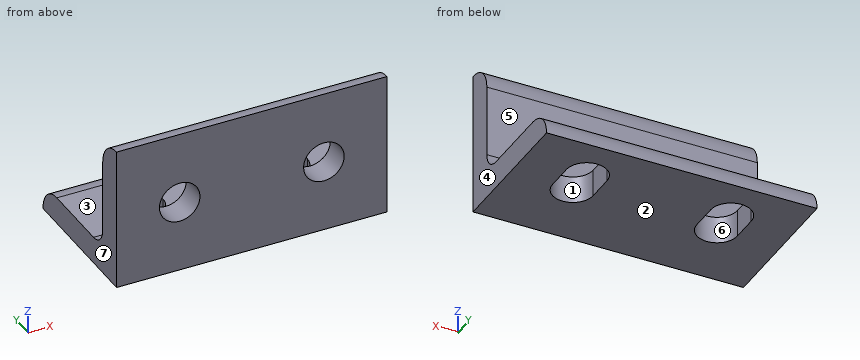
Autodesk Inventor part; units mm, degrees
ref_plane "YZ Plane" through (0, 0, 0) normal (1, 0, 0) x (0, 1, 0)
ref_plane "XZ Plane" through (0, 0, 0) normal (0, 1, 0) x (-1, 0, 0)
ref_plane "XY Plane" through (0, 0, 0) normal (0, 0, 1) x (1, 0, 0)
sketch "Sketch_1" plane through (0, 0, 0) normal (1, 0, 0) x (0, 1, 0)
  line L0 (0, 25.4) -> (0, 0)
  line L1 (0, 0) -> (25.4, 0)
  arc A0 (25.4, 0) -> (20.6248, 4.7752) centre (20.6248, 0) ccw
  line L2 (20.6248, 4.7752) -> (7.9502, 4.7752)
  arc A1 (4.7752, 7.9502) -> (7.9502, 4.7752) centre (7.9502, 7.9502) ccw
  line L3 (4.7752, 7.9502) -> (4.7752, 20.6248)
  arc A2 (4.7752, 20.6248) -> (0, 25.4) centre (0, 20.6248) ccw
extrude "Extrusion1" add sketch "Sketch_1" along normal mid plane 47.625
sketch "Sketch2" plane through (-23.8125, 0, 0) normal (0, -1, 0) x (1, 0, 0)
  point P0 (36.5125, 12.7)
hole "Hole1" at (12.7, 0, 12.7) direction (0, 1, 0) diameter 7.1374 depth 10.4648
sketch "Sketch3" plane through (-23.8125, 0, 0) normal (0, -1, 0) x (1, 0, 0)
  point P0 (11.1252, 12.7)
hole "Hole2" at (-12.6873, 0, 12.7) direction (0, 1, 0) diameter 7.1374 depth 10.4648
sketch "Sketch_2" plane through (0, 0, 0) normal (0, 0, 1) x (1, 0, 0)
  arc A0 (9.1313, 12.7) -> (16.2687, 12.7) centre (12.7, 12.7) ccw
  line L0 (16.2687, 12.7) -> (16.2687, 17.4752)
  arc A1 (16.2687, 17.4752) -> (9.1313, 17.4752) centre (12.7, 17.4752) ccw
  line L1 (9.1313, 17.4752) -> (9.1313, 12.7)
extrude "Extrusion2" cut sketch "Sketch_2" along normal blind 7.1628
sketch "Sketch_3" plane through (0, 0, 0) normal (0, 0, 1) x (1, 0, 0)
  arc A0 (-16.2687, 12.7) -> (-9.1313, 12.7) centre (-12.7, 12.7) ccw
  line L0 (-9.1313, 12.7) -> (-9.1313, 17.4752)
  arc A1 (-9.1313, 17.4752) -> (-16.2687, 17.4752) centre (-12.7, 17.4752) ccw
  line L1 (-16.2687, 17.4752) -> (-16.2687, 12.7)
extrude "Extrusion3" cut sketch "Sketch_3" along normal blind 7.1628
properties part number "4260"
Geometry: final body of the model. Coordinates: model frame, mm. Face numbers are marked on the shaded views. A direction names the side the tool comes from. Give positions to 0.01 mm unless a question says otherwise; leave off trailing zeros. Write each loop counter-clockwise with the first axis right and the second up, starting at its lowest first coordinate (ties: lowest second). Pieces come first, ordered by that corner, then holes.
(1) Cut plane C-C, the plane x = 7. Return loops of the section in (y, z) (3 decimals).
(2) Access query for the marked faces 1, 2 and 3. Directions: +Z, -Z, +X, -X, +Y, -Y. A direction counts if a zero-diameter tool reaches every point of the face in a straight line with its end or side. Return the directions, or none.
(3) First-contact query: P1, Ø9.5, axis at x = -12.69, z = 12.7, coming from the +Y side; P2, Ø11.5, axis at x = 12.7, z = 12.7, coming from the +Y side; P3, Ø5, axis at x = 13.5, z = 13, coming from the -Y side; P4, Ø3, axis at x = 14, y = 9, coming from the +Z side. Flat tips, straight axial feed; report the tip coordinate or a pass-through.
(4) Mould query, pull axis X, two halves, no side actions, for the marked faces 4, 5, 6 and 7. Classes: released by +X, released by -X, zero draft, split by the parting line, or undercut.
(5) Cut plane B-B, the plane y = 20. Return loops of the section in (x, z), then the cut area to 3 significant figures.
(6) Cut plane A-A, the plane z = 12.7. Return loops of the section in (x, y), then the cut area to 3 significant figures.
(7) Ray query, line 1 (X direction, y = 3, z = 12.7); line 2 (Z direction, x = 3.5, y = 10). Return the intervals inside material, ascending.
(8) Cut plane D-D, the plane x = 12.7. Return loops of the section in (y, z) (3 decimals).
Values follow:
1. outline: (0, 0) - (25.4, 0) arc R4.775 ccw to (20.625, 4.775) - (7.95, 4.775) arc R3.175 cw to (4.775, 7.95) - (4.775, 20.625) arc R4.775 ccw to (0, 25.4) - close
2. face 1: +Z, -Z
2. face 2: -Z, +X, -X, +Y, -Y
2. face 3: +Z, +X, -X, +Y
3. P1: stops at y = 4.78
3. P2: stops at y = 4.94
3. P3: passes through
3. P4: stops at z = 4.81
4. face 4: released by +X
4. face 5: zero draft
4. face 6: undercut
4. face 7: released by -X
5. outline: (-23.81, 0) - (-15.22, 0) - (-15.22, 4.78) - (-23.81, 4.78) - close; (-10.18, 0) - (10.18, 0) - (10.18, 4.78) - (-10.18, 4.78) - close; (15.22, 0) - (23.81, 0) - (23.81, 4.78) - (15.22, 4.78) - close
5. area: 179 mm2
6. outline: (-23.81, 0) - (-16.26, 0) - (-16.26, 4.78) - (-23.81, 4.78) - close; (-9.12, 0) - (9.13, 0) - (9.13, 4.78) - (-9.12, 4.78) - close; (16.27, 0) - (23.81, 0) - (23.81, 4.78) - (16.27, 4.78) - close
6. area: 159 mm2
7. line 1: x = -23.81 to -16.26, -9.12 to 9.13, 16.27 to 23.81
7. line 2: z = 0 to 4.78
8. outline: (0, 0) - (9.131, 0) - (9.131, 4.775) - (7.95, 4.775) arc R3.175 cw to (4.775, 7.95) - (4.775, 9.131) - (0, 9.131) - close; (0, 16.269) - (4.775, 16.269) - (4.775, 20.625) arc R4.775 ccw to (0, 25.4) - close; (21.044, 0) - (25.4, 0) arc R4.775 ccw to (21.044, 4.757) - close
